The model under review builds one solid part; all positions refer to its coordinate system, in mm. A direction names the side the tool comes from. Coordinates: 2 decimals unless noted, no trailing zeros. Loops run counter-clockwise (first coordinate to the right, second up) from the corner with the lowest first, then second, coordinate; pieces in that order, holes last. Notation, with made-up numbers: (76, -26) - (114, -26) arc R21 ccw to (114, -6) - close; hole circle Ø11 at (4.25, 65.5). An arc over 180 degrees is marked (long way). Answer in a Markdown table with one row per item. Add a question column.
(1) We need section C-C on z = -87. Write out the cut boundary in (x, y).
(2) For P1, Ø20, axis at x = 141.5, z = -806.5, coming from the -Y side; P2, Ø20, axis at x = 1073.5, z = -811.5, coming from the +Y side; P3, Ø20, axis at y = 381.5, z = -812, coming from the -X side, all flat-tipped, find the tip position at first contact; note any pin that passes through.
(3) We need section B-B on x = 1050. Write out the cut boundary in (y, z).
(4) We need section D-D on y = 400. Write out the cut boundary in (x, z), plus the area to 3 significant figures.
(5) Mouldability with a two-part tool opening along Z and no side actions: class faces 3 (the flat face through (194, 395, -800)), 4 (the flat face through (1049, 395, -825)), 5 (the flat face through (592, 406, 25)) as +Z half, -Z half, draft (parallel to the pull), parting line (faces both ways), or undercut.
(6) Machinability: for faces 1 (the flat face through (149, 395, -825)), 2 (the cylindrical face through (144.79, 360.34, -394.4)), which of the approach directions +Z, -Z, +X, -X, +Y, -Y give a long, thin tool a straight path to every point of the face, cutting with its end or side? Answer none if there is none.
(7) For line 1 along Z through (x, y) = (193, 689); line 2 along Z through (x, y) = (988.5, 757); line 3 along X through (y, z) = (413.5, -178), list the stretches that pass through material, from the lowest coordinate up.
(8) We need section A-A on y = 722. Write out the cut boundary in (x, z), plus the area to 3 significant figures.
from build123d import *

# Parameters (mm, degrees)
F0_W     = 1200
F0_H     = 800
F1_DEPTH = 25
F2_R     = 40
F3_DEPTH = 800
F4_W     = 100
F4_H     = 700
F5_DEPTH = 25
F6_W     = 100
F6_H     = 700
F7_DEPTH = 25
F8_R     = 25


with BuildPart() as f1:
    # F0 (on Top) → F1 (new body)
    with BuildSketch(Plane.XY):
        with Locations((600, 400)):
            Rectangle(F0_W, F0_H)
    extrude(amount=F1_DEPTH)

    # F2 (on face) → F3 (join)
    with BuildSketch(Plane(origin=(0, 0, 0), x_dir=(1, 0, 0), z_dir=(0, 0, -1))):
        with Locations((150, -400)):
            Circle(F2_R)
        with Locations((1050, -400)):
            Circle(F2_R)
    extrude(amount=F3_DEPTH)

    # F4 (on face) → F5 (join)
    with BuildSketch(Plane(origin=(0, 0, -800), x_dir=(1, 0, 0), z_dir=(0, 0, -1))):
        with Locations((150, -400)):
            Rectangle(F4_W, F4_H)
    extrude(amount=F5_DEPTH)

    # F6 (on face) → F7 (join)
    with BuildSketch(Plane(origin=(0, 0, -800), x_dir=(1, 0, 0), z_dir=(0, 0, -1))):
        with Locations((1050, -400)):
            Rectangle(F6_W, F6_H)
    extrude(amount=F7_DEPTH)

    # F8
    f8_edges = [f1.edges().sort_by_distance(p)[0] for p in [
        (1200, 0, 12.5),
        (1200, 800, 12.5),
        (0, 0, 12.5),
        (0, 800, 12.5),
    ]]
    fillet(f8_edges, radius=F8_R)


with BuildPart() as f9_1:
    # F9: copy of F1
    add(f1.part)


solid = f1.part
Outcome:
| question | item | result |
|---|---|---|
| 1 | outline | circle Ø80 at (150, 400); circle Ø80 at (1050, 400) |
| 2 | P1 | y = 50 |
| 2 | P2 | y = 750 |
| 2 | P3 | x = 100 |
| 3 | outline | (0, 0) - (360, 0) - (360, -800) - (50, -800) - (50, -825) - (750, -825) - (750, -800) - (440, -800) - (440, 0) - (800, 0) - (800, 25) - (0, 25) - close |
| 4 | outline | (0, 0) - (110, 0) - (110, -800) - (100, -800) - (100, -825) - (200, -825) - (200, -800) - (190, -800) - (190, 0) - (1010, 0) - (1010, -800) - (1000, -800) - (1000, -825) - (1100, -825) - (1100, -800) - (1090, -800) - (1090, 0) - (1200, 0) - (1200, 25) - (0, 25) - close |
| 4 | area | 163,000 mm² |
| 5 | face 3 | undercut |
| 5 | face 4 | -Z half |
| 5 | face 5 | +Z half |
| 6 | face 1 | -Z, +X, -X, +Y, -Y |
| 6 | face 2 | none |
| 7 | line 1 | -825 to -800, 0 to 25 |
| 7 | line 2 | 0 to 25 |
| 7 | line 3 | 112.35 to 187.65, 1012.35 to 1087.65 |
| 8 | outline | (0, 0) - (1200, 0) - (1200, 25) - (0, 25) - close; (100, -825) - (200, -825) - (200, -800) - (100, -800) - close; (1000, -825) - (1100, -825) - (1100, -800) - (1000, -800) - close |
| 8 | area | 35,000 mm² |
